For this review, take the finished solid that the model builds, in its own axes (mm). A direction names the side the tool comes from. Give positions to 0.01 mm unless a question says otherwise; leave off trailing zeros. Order: outer loops, then holes, each group sorted by start corner. A loop starts at its lowest first (then second) coordinate and runs counter-clockwise, first axis right, second up.
from build123d import *

# Parameters (mm, degrees)
SKETCH1_W             = 41
SKETCH1_H             = 36
BOSS_EXTRUDE1_DEPTH   = 20
BOSS_EXTRUDE2_DEPTH   = 2
BOSS_EXTRUDE3_DEPTH   = 1.9
SKETCH3_R             = 6.5
SKETCH3_R_2           = 5.5
BOSS_EXTRUDE4_DEPTH   = 1.5
SKETCH3_3_R           = 5.5
SKETCH3_3_R_2         = 3
BOSS_EXTRUDE5_DEPTH   = 2
SKETCH10_R            = 0.825
CUT_EXTRUDE3_DEPTH    = 1.5
SKETCH10_10_R         = 0.825
CUT_EXTRUDE4_DEPTH    = 32
CHAMFER2_SIZE         = 2.5
CHAMFER2_SIZE2        = 0.909925586
CHAMFER2_PART_2_SIZE  = 2.5
CHAMFER2_PART_2_SIZE2 = 0.909925586
CHAMFER2_PART_3_SIZE  = 2.5
CHAMFER2_PART_3_SIZE2 = 0.909925586
CHAMFER2_PART_4_SIZE  = 2.5
CHAMFER2_PART_4_SIZE2 = 0.909925586
FILLET2_R             = 0.5
SKETCH11_W            = 7.5
SKETCH11_H            = 4.1
BOSS_EXTRUDE10_DEPTH  = 7
BOSS_EXTRUDE10_TAPER  = 5


with BuildPart() as part:
    # Sketch1 → Boss-Extrude1 (new body)
    with BuildSketch(Plane(origin=(0, 0, 0), x_dir=(0, 0, -1), z_dir=(1, 0, 0))):
        Rectangle(SKETCH1_W, SKETCH1_H)
    extrude(amount=BOSS_EXTRUDE1_DEPTH)

    # Sketch2 → Boss-Extrude2 (add)
    with BuildSketch(Plane(origin=(0, 18, 0), x_dir=(1, 0, 0), z_dir=(0, 1, 0))):
        with BuildLine():
            ThreePointArc((20, 10.4), (7.763932023, 20.146794345), (1, 6.041101056))
            Line((1, 6.041101056), (1, 10.5))
            Line((1, 10.5), (19, 10.5))
            Line((19, 10.5), (19, 6.041101056))
            ThreePointArc((19, 6.041101056), (19.746794345, 8.163932022), (20, 10.4))
        make_face()
        with BuildLine():
            Line((1, 10.5), (1, 6.041101056))
            ThreePointArc((1, 6.041101056), (10, 0.4), (19, 6.041101056))
            Line((19, 6.041101056), (19, 10.5))
            Line((19, 10.5), (1, 10.5))
        make_face()
        with BuildLine():
            Line((1, 6.041101056), (1, -14.5))
            Line((1, -14.5), (5.25, -14.5))
            Line((5.25, -14.5), (14.75, -14.5))
            Line((14.75, -14.5), (19, -14.5))
            Line((19, -14.5), (19, 6.041101056))
            ThreePointArc((19, 6.041101056), (10, 0.4), (1, 6.041101056))
        make_face()
    extrude(amount=BOSS_EXTRUDE2_DEPTH)

    # Sketch2<3> → Boss-Extrude3 (add)
    with BuildSketch(Plane(origin=(0, 18, 0), x_dir=(1, 0, 0), z_dir=(0, 1, 0))):
        with BuildLine():
            Line((14.75, -14.5), (5.25, -14.5))
            ThreePointArc((5.25, -14.5), (10, -17), (14.75, -14.5))
        make_face()
    extrude(amount=BOSS_EXTRUDE3_DEPTH)

    # Sketch3 → Boss-Extrude4 (add)
    with BuildSketch(Plane(origin=(0, 20, 0), x_dir=(1, 0, 0), z_dir=(0, 1, 0))):
        with Locations(Location((10, 10.4, 0), (0, 0, 270))):
            Circle(SKETCH3_R)
        with Locations(Location((10, 10.4, 0), (0, 0, 270))):
            Circle(SKETCH3_R_2, mode=Mode.SUBTRACT)
    extrude(amount=BOSS_EXTRUDE4_DEPTH)

    # Sketch3<3> → Boss-Extrude5 (add)
    with BuildSketch(Plane(origin=(0, 20, 0), x_dir=(1, 0, 0), z_dir=(0, 1, 0))):
        with Locations(Location((10, 10.4, 0), (0, 0, 270))):
            Circle(SKETCH3_3_R)
        with Locations(Location((10, 10.4, 0), (0, 0, 270))):
            Circle(SKETCH3_3_R_2, mode=Mode.SUBTRACT)
    extrude(amount=BOSS_EXTRUDE5_DEPTH)

    # Sketch10 → Cut-Extrude3 (cut)
    # profile 1 of 4: a face of its own
    with BuildSketch(Plane.XZ.offset(18)):
        with BuildLine():
            Line((0, 16.65), (2.5, 16.65))
            ThreePointArc((2.5, 16.65), (3.808147545, 17.191852455), (4.35, 18.5))
            Line((4.35, 18.5), (4.35, 20.5))
            Line((4.35, 20.5), (0, 20.5))
            Line((0, 20.5), (0, 16.65))
        make_face()
        with Locations(Location((2.5, 18.5, 0), (0, 0, 270))):
            Circle(SKETCH10_R, mode=Mode.SUBTRACT)
    # profile 2 of 4: a face of its own
    with BuildSketch(Plane.XZ.offset(18)):
        with BuildLine():
            Line((15.65, 18.5), (15.65, 20.5))
            Line((15.65, 20.5), (20, 20.5))
            Line((20, 20.5), (20, 16.65))
            Line((20, 16.65), (17.5, 16.65))
            ThreePointArc((17.5, 16.65), (16.191852455, 17.191852455), (15.65, 18.5))
        make_face()
        with Locations(Location((17.5, 18.5, 0), (0, 0, 90))):
            Circle(SKETCH10_R, mode=Mode.SUBTRACT)
    # profile 3 of 4: a face of its own
    with BuildSketch(Plane.XZ.offset(18)):
        with BuildLine():
            Line((4.35, -18.5), (4.35, -20.5))
            Line((4.35, -20.5), (0, -20.5))
            Line((0, -20.5), (0, -16.65))
            Line((0, -16.65), (2.5, -16.65))
            ThreePointArc((2.5, -16.65), (3.808147545, -17.191852455), (4.35, -18.5))
        make_face()
        with Locations(Location((2.5, -18.5, 0), (0, 0, 90))):
            Circle(SKETCH10_R, mode=Mode.SUBTRACT)
    # profile 4 of 4: a face of its own
    with BuildSketch(Plane.XZ.offset(18)):
        with BuildLine():
            Line((20, -16.65), (17.5, -16.65))
            ThreePointArc((17.5, -16.65), (16.191852455, -17.191852455), (15.65, -18.5))
            Line((15.65, -18.5), (15.65, -20.5))
            Line((15.65, -20.5), (20, -20.5))
            Line((20, -20.5), (20, -16.65))
        make_face()
        with Locations(Location((17.5, -18.5, 0), (0, 0, 270))):
            Circle(SKETCH10_R, mode=Mode.SUBTRACT)
    extrude(amount=-CUT_EXTRUDE3_DEPTH, mode=Mode.SUBTRACT)

    # Sketch10<10> → Cut-Extrude4 (cut)
    with BuildSketch(Plane.XZ.offset(18)):
        with Locations(Location((2.5, 18.5, 0), (0, 0, 270))):
            Circle(SKETCH10_10_R)
        with Locations(Location((17.5, 18.5, 0), (0, 0, 270))):
            Circle(SKETCH10_10_R)
        with Locations(Location((17.5, -18.5, 0), (0, 0, 270))):
            Circle(SKETCH10_10_R)
        with Locations(Location((2.5, -18.5, 0), (0, 0, 270))):
            Circle(SKETCH10_10_R)
    extrude(amount=-CUT_EXTRUDE4_DEPTH, mode=Mode.SUBTRACT)

    # Chamfer2
    chamfer2_edges = [part.edges().sort_by_distance(p)[0] for p in [
        (10, -18, 20.5),
    ]]
    chamfer2_side = [part.faces().sort_by_distance(p)[0] for p in [
        (10, 0.318427753, 20.5),
    ]]
    chamfer(chamfer2_edges, length=CHAMFER2_SIZE, length2=CHAMFER2_SIZE2, reference=chamfer2_side[0])

    # Chamfer2 part 2
    chamfer2_part_2_edges = [part.edges().sort_by_distance(p)[0] for p in [
        (20, -18, 0),
    ]]
    chamfer2_part_2_side = [part.faces().sort_by_distance(p)[0] for p in [
        (20, 0.13604937, 0),
    ]]
    chamfer(chamfer2_part_2_edges, length=CHAMFER2_PART_2_SIZE, length2=CHAMFER2_PART_2_SIZE2, reference=chamfer2_part_2_side[0])

    # Chamfer2 part 3
    chamfer2_part_3_edges = [part.edges().sort_by_distance(p)[0] for p in [
        (10, -18, -20.5),
    ]]
    chamfer2_part_3_side = [part.faces().sort_by_distance(p)[0] for p in [
        (10, 0.318427753, -20.5),
    ]]
    chamfer(chamfer2_part_3_edges, length=CHAMFER2_PART_3_SIZE, length2=CHAMFER2_PART_3_SIZE2, reference=chamfer2_part_3_side[0])

    # Chamfer2 part 4
    chamfer2_part_4_edges = [part.edges().sort_by_distance(p)[0] for p in [
        (0, -18, 0),
    ]]
    chamfer2_part_4_side = [part.faces().sort_by_distance(p)[0] for p in [
        (0, 0.13604937, 0),
    ]]
    chamfer(chamfer2_part_4_edges, length=CHAMFER2_PART_4_SIZE, length2=CHAMFER2_PART_4_SIZE2, reference=chamfer2_part_4_side[0])

    # Fillet2
    # the kernel refuses this fillet: 0.5 mm, written as the material it takes off along each edge
    with BuildSketch(Plane(origin=(20, 19.25, 20.5), x_dir=(-1, 0, 0), z_dir=(0, -1, 0)), Plane(origin=(0, -16.75, -20.5), x_dir=(0, 0, 1), z_dir=(0, 1, 0)), Plane(origin=(20, -16.75, -20.5), x_dir=(-1, 0, 0), z_dir=(0, 1, 0)), Plane(origin=(0, 19.25, 20.5), x_dir=(0, 0, -1), z_dir=(0, -1, 0))) as fillet2_piece_1:
        with BuildLine():
            CenterArc((FILLET2_R, FILLET2_R), FILLET2_R, 180, 90)
            Line((0, FILLET2_R), (0, 0))
            Line((0, 0), (FILLET2_R, 0))
        make_face()
    extrude(amount=36, mode=Mode.SUBTRACT)
    with BuildSketch(Plane(origin=(19.090074414, -18, 17.525259423), x_dir=(-1, 0, 0), z_dir=(0, 0, -1))) as fillet2_piece_2:
        with BuildLine():
            CenterArc((FILLET2_R * 0.70020753821, FILLET2_R), FILLET2_R, 200, 70)
            Line((-FILLET2_R * 0.239485082576, FILLET2_R * 0.657979856674), (0, 0))
            Line((0, 0), (FILLET2_R * 0.70020753821, 0))
        make_face()
    extrude(amount=35.050518846, mode=Mode.SUBTRACT)
    with BuildSketch(Plane(origin=(3.474740577, -18, 19.590074414), x_dir=(0, 0, -1), z_dir=(1, 0, 0))) as fillet2_piece_3:
        with BuildLine():
            CenterArc((FILLET2_R * 0.70020753821, FILLET2_R), FILLET2_R, 200, 70)
            Line((-FILLET2_R * 0.239485082576, FILLET2_R * 0.657979856674), (0, 0))
            Line((0, 0), (FILLET2_R * 0.70020753821, 0))
        make_face()
    extrude(amount=13.050518846, mode=Mode.SUBTRACT)
    with BuildSketch(Plane(origin=(0.909925586, -18, 17.525259423), x_dir=(1, 0, 0), z_dir=(0, 0, -1))) as fillet2_piece_4:
        with BuildLine():
            CenterArc((FILLET2_R * 0.70020753821, -FILLET2_R), FILLET2_R, 90, 70)
            Line((-FILLET2_R * 0.239485082576, -FILLET2_R * 0.657979856674), (0, 0))
            Line((0, 0), (FILLET2_R * 0.70020753821, 0))
        make_face()
    extrude(amount=35.050518846, mode=Mode.SUBTRACT)
    with BuildSketch(Plane(origin=(3.474740577, -18, -19.590074414), x_dir=(0, 0, 1), z_dir=(1, 0, 0))) as fillet2_piece_5:
        with BuildLine():
            CenterArc((FILLET2_R * 0.70020753821, -FILLET2_R), FILLET2_R, 90, 70)
            Line((-FILLET2_R * 0.239485082576, -FILLET2_R * 0.657979856674), (0, 0))
            Line((0, 0), (FILLET2_R * 0.70020753821, 0))
        make_face()
    extrude(amount=13.050518846, mode=Mode.SUBTRACT)
    with BuildSketch(Plane(origin=(20.359668978, -14.511817604, 20.859668978), x_dir=(-0.9461886483394649, 0.3040991697893318, 0.1106830460683808), z_dir=(-0.3236155771181854, -0.8891264907159879, -0.3236155771181854)), Plane(origin=(-0.359668978, -14.511817604, 20.859668978), x_dir=(-0.11068304606838054, 0.30409916978933194, -0.9461886483394649), z_dir=(0.3236155771181852, -0.8891264907159879, -0.32361557711818534))) as fillet2_piece_6:
        with BuildLine():
            CenterArc((FILLET2_R * 0.889126490716, FILLET2_R), FILLET2_R, 186.717713464, 83.282286536)
            Line((-FILLET2_R * 0.104008041637, FILLET2_R * 0.883022221559), (0, 0))
            Line((0, 0), (FILLET2_R * 0.889126490716, 0))
        make_face()
    extrude(amount=3.347515592, mode=Mode.SUBTRACT)
    with BuildSketch(Plane(origin=(20.359668978, -14.511817604, -20.859668978), x_dir=(-0.9461886483394651, 0.3040991697893314, -0.1106830460683821), z_dir=(-0.3236155771181854, -0.8891264907159879, 0.3236155771181854)), Plane(origin=(-0.359668978, -14.511817604, -20.859668978), x_dir=(-0.11068304606838054, 0.30409916978933194, 0.946188648339465), z_dir=(0.3236155771181852, -0.8891264907159879, 0.32361557711818534))) as fillet2_piece_7:
        with BuildLine():
            CenterArc((FILLET2_R * 0.889126490716, -FILLET2_R), FILLET2_R, 90, 83.282286536)
            Line((-FILLET2_R * 0.104008041637, -FILLET2_R * 0.883022221559), (0, 0))
            Line((0, 0), (FILLET2_R * 0.889126490716, 0))
        make_face()
    extrude(amount=3.347515592, mode=Mode.SUBTRACT)

    # Sketch11 → Boss-Extrude10 (add)
    with BuildSketch(Plane(origin=(0, 0, -20.5), x_dir=(-1, 0, 0), z_dir=(0, 0, -1))):
        with Locations((-10, -11.45)):
            Rectangle(SKETCH11_W, SKETCH11_H)
    extrude(amount=BOSS_EXTRUDE10_DEPTH, taper=BOSS_EXTRUDE10_TAPER)


solid = part.part
1) Clearance check with flat-ended pins moving along their axes: pin 1 (1.9 mm diameter, centred on x = 17.5, z = -18.5, fed in from +Y); pin 2 (1.7 mm diameter, centred on x = 2, z = -18.5, fed in from -Y); pin 3 (3.5 mm diameter, centred on x = 10, z = -10.4, fed in from +Y). State where each tip first meets the part, or that it passes through.
Answer sheet:
pin 1: stops at y = 18
pin 2: stops at y = -16.5
pin 3: stops at y = 20
2) Draft analysis for pull direction X (two halves, no side actions). For faces 1 (the face through (7.89, 21.75, -5.32)), 2 (the face through (19, -16.5, -18)), 3 (the face through (17.5, 14, 18.5)), state which applies: +X half, -X half, draft (parallel to the pull), parting line (faces both ways), or undercut.
Answer sheet:
face 1: parting line
face 2: draft
face 3: undercut
3) We need section A-A on y = 4. Give the boundary of the cut face in (x, z) (3 decimals), then the cut area to 3 significant figures.
Answer sheet:
outline: (0, -20) arc R0.5 ccw to (0.5, -20.5) - (19.5, -20.5) arc R0.5 ccw to (20, -20) - (20, 20) arc R0.5 ccw to (19.5, 20.5) - (0.5, 20.5) arc R0.5 ccw to (0, 20) - close; hole circle Ø1.65 at (2.5, -18.5); hole circle Ø1.65 at (2.5, 18.5); hole circle Ø1.65 at (17.5, -18.5); hole circle Ø1.65 at (17.5, 18.5)
area: 811 mm2
4) To check wall thickness, follow line 1 (X direction, y = -5, z = -18.5) (3 decimals); line 2 (Z direction, x = 3, y = -13); line 3 (X direction, y = 4, z = 18). State the ranges of each line that lie inside material, in increasing order.
Answer sheet:
line 1: x = 0 to 1.675, 3.325 to 16.675, 18.325 to 20
line 2: z = -20.5 to -19.16, -17.84 to 17.84, 19.16 to 20.5
line 3: x = 0 to 1.84, 3.16 to 16.84, 18.16 to 20
5) Tool access review of faces 4 (the face through (11.95, 20.74, -4.2)), 5 (the face through (2, -17, -16.65)), 6 (the face through (10, 19.9, 15)), 7 (the face through (2.536, -1.463, 19.324)), 8 (the face through (3.794, -17.26, 17.178)): name each direction out of +Z, -Z, +X, -X, +Y, -Y from which nothing blocks a thin tool from reaching the whole face with its end or side.
Answer sheet:
face 4: +Y
face 5: -Z, -X, -Y
face 6: +Z, +X, -X, +Y
face 7: -Y
face 8: +Z, -X, -Y
